from build123d import *

# Parameters (mm, degrees)
ESQUISSE1_W             = 90.6
ESQUISSE1_H             = 10
BOSS_EXTRU_1_DEPTH      = 10
ESQUISSE2_W             = 90.6
ESQUISSE2_H             = 4
ENL_V_MAT_EXTRU_1_DEPTH = 6
ESQUISSE3_R             = 1.4
ENL_V_MAT_EXTRU_2_DEPTH = 6
ESQUISSE4_W             = 50
ESQUISSE4_H             = 1.8
BOSS_EXTRU_2_DEPTH      = 1.5
ESQUISSE5_R             = 2.75
ENL_V_MAT_EXTRU_3_DEPTH = 4
ESQUISSE6_R             = 1.4
ENL_V_MAT_EXTRU_4_DEPTH = 11


with BuildPart() as part:
    # Esquisse1 → Boss.-Extru.1 (new body)
    with BuildSketch(Plane.XY):
        with Locations((45.3, 5)):
            Rectangle(ESQUISSE1_W, ESQUISSE1_H)
    extrude(amount=BOSS_EXTRU_1_DEPTH)

    # Esquisse2 → Enlèv. mat.-Extru.1 (cut)
    with BuildSketch(Plane.XY.offset(10)):
        with Locations((45.3, 8)):
            Rectangle(ESQUISSE2_W, ESQUISSE2_H)
    extrude(amount=-ENL_V_MAT_EXTRU_1_DEPTH, mode=Mode.SUBTRACT)

    # Esquisse3 → Enlèv. mat.-Extru.2 (cut)
    with BuildSketch(Plane(origin=(0, 6, 0), x_dir=(1, 0, 0), z_dir=(0, 1, 0))):
        with Locations((6.65, -5.5)):
            Circle(ESQUISSE3_R)
        with Locations((83.95, -6.5)):
            Circle(ESQUISSE3_R)
    extrude(amount=-ENL_V_MAT_EXTRU_2_DEPTH, mode=Mode.SUBTRACT)

    # Esquisse4 → Boss.-Extru.2 (add)
    with BuildSketch(Plane.XY.offset(4)):
        with Locations((45.3, 9.1)):
            Rectangle(ESQUISSE4_W, ESQUISSE4_H)
    extrude(amount=BOSS_EXTRU_2_DEPTH)

    # Esquisse5 → Enlèv. mat.-Extru.3 (cut)
    with BuildSketch(Plane(origin=(0, 10, 0), x_dir=(1, 0, 0), z_dir=(0, 1, 0))):
        with Locations((6.65, -5.5)):
            Circle(ESQUISSE5_R)
        with Locations((83.95, -6.5)):
            Circle(ESQUISSE5_R)
    extrude(amount=-ENL_V_MAT_EXTRU_3_DEPTH, mode=Mode.SUBTRACT)

    # Esquisse6 → Enlèv. mat.-Extru.4 (cut, through all)
    with BuildSketch(Plane.XY.offset(10)):
        with Locations((20.3, 3)):
            Circle(ESQUISSE6_R)
        with Locations((70.3, 3)):
            Circle(ESQUISSE6_R)
    extrude(amount=-ENL_V_MAT_EXTRU_4_DEPTH, mode=Mode.SUBTRACT)


solid = part.part
Design review of the part built by this model. Coordinates are the model's own, in mm. A direction names the side the tool comes from. Give positions to 0.01 mm unless a question says otherwise; leave off trailing zeros. Loops run counter-clockwise (first coordinate to the right, second up) from the corner with the lowest first, then second, coordinate; pieces in that order, holes last. Notation, with made-up numbers: (-10, -17) - (25, -17) arc R22 cw to (25, 20) - close; hole circle Ø6 at (89.5, 84). An arc over 180 degrees is marked (long way). Write item = value, one per line.
1) Clearance check with flat-ended pins moving along their axes: pin 1 Ø3.5 at (x, z) = (83.95, 6.5) entering from +Y; pin 2 Ø2 at (x, y) = (3, 7.5) entering from +Z; pin 3 Ø3 at (x, y) = (56, 8.5) entering from +Z; pin 4 Ø1.7 at (x, z) = (6.65, 5.5) entering from +Y. State where each tip first meets the part, or that it passes through.
Result sheet:
pin_1 = 6
pin_2 = 4
pin_3 = 5.5
pin_4 = through
2) Take a section at A-A on y = 3. State the section outline as (x, z) points, and give its area (3 significant figures).
Result sheet:
outline = (0, 0) - (18.9, 0) - (18.9, 10) - (0, 10) - close; (21.7, 0) - (68.9, 0) - (68.9, 10) - (21.7, 10) - close; (71.7, 0) - (90.6, 0) - (90.6, 10) - (71.7, 10) - close; hole circle Ø2.8 at (6.65, 5.5); hole circle Ø2.8 at (83.95, 6.5)
area = 838 mm2
3) Take a section at C-C on x = 31. State the section outline as (y, z) points.
Result sheet:
outline = (0, 0) - (10, 0) - (10, 5.5) - (8.2, 5.5) - (8.2, 4) - (6, 4) - (6, 10) - (0, 10) - close
4) Take a section at D-D on x = 83.95. State the section outline as (y, z) points.
Result sheet:
outline = (0, 0) - (10, 0) - (10, 3.75) - (6, 3.75) - (6, 5.1) - (0, 5.1) - close; (0, 7.9) - (6, 7.9) - (6, 10) - (0, 10) - close
5) Tool access review of faces 4 (the face through (45, 8.2, 5)), 5 (the face through (70.3, 9, 5)), 6 (the face through (2, 8, 4)), 7 (the face through (83.97, 8.03, 3.75)): name each direction out of +Z, -Z, +X, -X, +Y, -Y from which nothing blocks a thin tool from reaching the whole face with its end or side.
Result sheet:
face_4 = +Z, +X, -X
face_5 = +Z, +X, +Y
face_6 = +Z, -X, +Y
face_7 = +Z, +Y
6) Draft analysis for pull direction X (two halves, no side actions). For faces 1 (the face through (88, 8, 4)), 2 (the face through (6.69, 8.03, 2.75)), 3 (the face through (0, 4, 4)), state which applies: +X half, -X half, draft (parallel to the pull), parting line (faces both ways), or undercut.
Result sheet:
face_1 = draft
face_2 = undercut
face_3 = -X half
7) Take a section at B-B on x = 6.65. State the section outline as (y, z) points.
Result sheet:
outline = (0, 0) - (10, 0) - (10, 2.75) - (6, 2.75) - (6, 4.1) - (0, 4.1) - close; (0, 6.9) - (6, 6.9) - (6, 10) - (0, 10) - close
8) To check wall thickness, follow line 1 (Z direction, x = 6.65, y = 1.9); line 2 (Y direction, x = 20.3, z = 7); line 3 (X direction, y = 3.25, z = 1.5). State the ranges of each line that lie inside material, in increasing order.
Result sheet:
line_1 = 0 to 4.1, 6.9 to 10
line_2 = 0 to 1.6, 4.4 to 6
line_3 = 0 to 18.92, 21.68 to 68.92, 71.68 to 90.6
